Autodesk Inventor part; units mm, degrees
ref_plane "Work Plane1" through (-5, 0, -50) normal (0, 0, 1) x (1, 0, 0)
ref_plane "YZ Plane" through (0, 0, 0) normal (1, 0, 0) x (0, 1, 0)
ref_plane "XZ Plane" through (0, 0, 0) normal (0, 1, 0) x (-1, 0, 0)
sketch "Sketch2" plane through (0, 0, 0) normal (0, 1, 0) x (-1, 0, 0)
  line L0 (0, 0) -> (5, 0)
  line L1 (5, 0) -> (5, -100)
  line L2 (5, -100) -> (0, -100)
  line L3 (0, -100) -> (0, 0)
  dimension "d0" = 5
  dimension "d1" = 100
extrude "Extrusion1" add sketch "Sketch2" along normal blind 75
sketch "Sketch5" plane through (0, 0, 0) normal (1, 0, 0) x (0, 0, -1)
  line L0 (0, 75) -> (100, 75)
  line L1 (22, 23.95) -> (42, 23.95)
  line L2 (42, 23.95) -> (42, 75)
  line L3 (42, 75) -> (22, 75)
  line L4 (22, 75) -> (22, 23.95)
  line L5 (58, 23.95) -> (78, 23.95)
  line L6 (78, 23.95) -> (78, 75)
  line L7 (78, 75) -> (58, 75)
  line L8 (58, 75) -> (58, 23.95)
  line L9 (0, 0) -> (0, 75)
  line L10 (100, 0) -> (100, 75)
  line L11 (100, 0) -> (0, 0)
  dimension "d16" = 16
  dimension "d17" = 22
  dimension "d18" = 22
  dimension "d20" = 23.95
extrude "Extrusion4" cut sketch "Sketch5" against normal through all contours L0 L2 L1 L4 | L0 L6 L5 L8
sketch "Sketch6" plane through (0, 0, 0) normal (1, 0, 0) x (0, 0, -1)
  line L0 (58, 23.95) -> (58, 75)
  line L1 (42, 5) -> (58, 5)
  line L2 (58, 5) -> (58, 75)
  line L3 (58, 75) -> (42, 75)
  line L4 (42, 75) -> (42, 5)
  line L5 (42, 75) -> (42, 23.95)
  point P0 (0, 0)
  dimension "d26" = 70
extrude "Extrusion5" cut sketch "Sketch6" against normal through all
sketch "Sketch7" plane through (0, 0, 0) normal (0, -1, 0) x (1, 0, 0)
  circle A0 centre (-2.5, -10) radius 1.5
  line L0 (0, 0) -> (-5, 0)
  line L1 (-5, 0) -> (-5, -100)
  dimension "d27" = 3
  dimension "d28" = 10
  dimension "d29" = 2.5
extrude "Extrusion6" add sketch "Sketch7" along normal blind 5
pattern_linear "Rectangular Pattern1" count 5 spacing 20 along (0, 0, -1) of "Extrusion6"
ref_plane "Work Plane1" through (-5, 0, -50) normal (0, 0, 1) x (1, 0, 0)
sketch "Sketch9" plane through (-5, -6.2824, -100) normal (-1, 0, 0) x (0, 0, 1)
  line L0 (100, 6.2824) -> (100, 75)
  line L1 (0, 29.2824) -> (100, 29.2824)
  line L2 (100, 29.2824) -> (100, 34.2824)
  line L3 (100, 34.2824) -> (0, 34.2824)
  line L4 (0, 34.2824) -> (0, 29.2824)
  circle A0 centre (92.5, 31.7824) radius 1.5
  line L5 (78, 75) -> (78, 23.95)
  line L6 (100, 75) -> (78, 75)
  line L7 (100, 6.2824) -> (95, 6.2824)
  line L8 (95, 6.2824) -> (95, 75)
  line L9 (95, 75) -> (100, 75)
  line L10 (100, 75) -> (100, 6.2824)
  line L11 (0, 75) -> (22, 75)
  line L12 (0, 0) -> (5, 0)
  line L13 (5, 0) -> (5, 75)
  line L14 (5, 75) -> (0, 75)
  line L15 (0, 75) -> (0, 0)
  point P0 (97.5, 6.2824)
  point P1 (100, 6.2824)
  dimension "d59" = 5
  dimension "d56" = 3
  dimension "d55" = 5
  dimension "d53" = 5
  dimension "d57" = 2.5
  dimension "d54" = 2.5
  dimension "d66" = 23
extrude "Extrusion8" cut sketch "Sketch9" against normal blind 2.5 contours A0
pattern_linear "Rectangular Pattern3" count 3 spacing 6 along (0, 0, -1) of "Extrusion8"
mirror "Mirror2" about plane through (-5, 0, -50) normal (0, 0, 1) of "Extrusion8", "Rectangular Pattern3"
sketch "Sketch10" plane through (-5, 0, -100) normal (-1, 0, 0) x (0, 0, 1)
  line L0 (78, 75) -> (100, 75)
  line L1 (100, 0) -> (95, 0)
  line L2 (95, 0) -> (95, 75)
  line L3 (95, 75) -> (100, 75)
  line L4 (100, 75) -> (100, 0)
  circle A0 centre (97.5, 7.5) radius 1.5
  dimension "d67" = 5
  dimension "d68" = 3
  dimension "d69" = 2.5
  dimension "d70" = 7.5
extrude "Extrusion9" cut sketch "Sketch10" against normal blind 2.5 contours A0
pattern_linear "Rectangular Pattern4" count 3 spacing 30 along (0, 1, 0) of "Extrusion9"
mirror "Mirror3" about plane through (-5, 0, -50) normal (0, 0, 1) of "Extrusion9", "Rectangular Pattern4"
properties part number "Back Plate V3"
Here's how the part is built. I have some questions about the finished solid (model axes, mm). A direction names the side the tool comes from. Give positions to 0.01 mm unless a question says otherwise; leave off trailing zeros. Write each loop counter-clockwise with the first axis right and the second up, starting at its lowest first coordinate (ties: lowest second). Pieces come first, ordered by that corner, then holes. Notation, with made-up numbers: (68, -19.5) -> (77, -19.5) arc R17 cw to (77, 11.5) -> close; hole circle Ø7 at (59.5, -21.75). An arc over 180 degrees is marked (long way). Use one line per item in the form item = value. Start each with the question number.
1. Will these pins go through, and if not, where does the flat tip stop? pin 1 Ø1.5 at (y, z) = (26, -80.5) entering from -X; pin 2 Ø3.5 at (y, z) = (25.5, -7.5) entering from +X.
2. Imagine slicing it at D-D on z = -30. List the corners of the cut face in (x, y) for me, plus the area to 3 significant figures.
3. Imagine slicing it at B-B on z = -97.5. List the corners of the cut face in (x, y) for me, plus the area to 4 significant figures.
4. Imagine slicing it at C-C on y = 22. List the corners of the cut face in (x, z) for me, plus the area to 3 significant figures.
5. Thinking about a two-plate mould opening in Y: for faces 1 (the face through (-2, 23.95, -68)), 2 (the face through (-3.768, 36.036, -2.825)), 3 (the face through (-2, 37, 0)), which applies, +Y half, -Y half, draft (parallel to the pull), parting line (faces both ways), or undercut?
6. Imagine slicing it at A-A on y = 41.5. List the corners of the cut face in (x, z) for me, plus the area to 3 significant figures.
7. If I drill on L1, parallel to Y at x = -3.85, z = -97.5; L2, parallel to Y at x = -4.35, z = -92.5; L3, parallel to Z at x = -3.1, y = 34, over which ranges is the centre line in solid material (lowest first)?
8. On a 3-axis mill with a long thin cutter (end or side, diameter ignored), from which of +Z, -Z, +X, -X, +Y, -Y can I reach the whole of each face in a straight line? I mean faces 4 (the face through (-2.825, -2.465, -48.536)), 5 (the face through (-3, -5, -70)), 6 (the face through (-2.5, 26, -20)), 7 (the face through (-2, 15, -42)). Say none if no direction works.
Entries:
q1.pin_1 = -2.5
q1.pin_2 = 0
q2.outline = (-5, 0) -> (-4, 0) -> (-4, -5) -> (-1, -5) -> (-1, 0) -> (0, 0) -> (0, 23.95) -> (-5, 23.95) -> close
q2.area = 135 mm²
q3.outline = (-5, 0) -> (0, 0) -> (0, 75) -> (-5, 75) -> (-5, 69) -> (-2.5, 69) -> (-2.5, 66) -> (-5, 66) -> (-5, 39) -> (-2.5, 39) -> (-2.5, 36) -> (-5, 36) -> (-5, 9) -> (-2.5, 9) -> (-2.5, 6) -> (-5, 6) -> close
q3.area = 352.5 mm²
q4.outline = (-5, -100) -> (0, -100) -> (0, -58) -> (-5, -58) -> close; (-5, -42) -> (0, -42) -> (0, 0) -> (-5, 0) -> close
q4.area = 420 mm²
q5.face_1 = +Y half
q5.face_2 = undercut
q5.face_3 = draft
q6.outline = (-5, -100) -> (0, -100) -> (0, -78) -> (-5, -78) -> close; (-5, -22) -> (0, -22) -> (0, 0) -> (-5, 0) -> close
q6.area = 220 mm²
q7.L1 = 0 to 6, 9 to 36, 39 to 66, 69 to 75
q7.L2 = 0 to 24, 27 to 75
q7.L3 = -100 to -78, -22 to 0
q8.face_4 = -Y
q8.face_5 = +Z, -Z, +X, -X, -Y
q8.face_6 = -X
q8.face_7 = +X, -X, +Y
